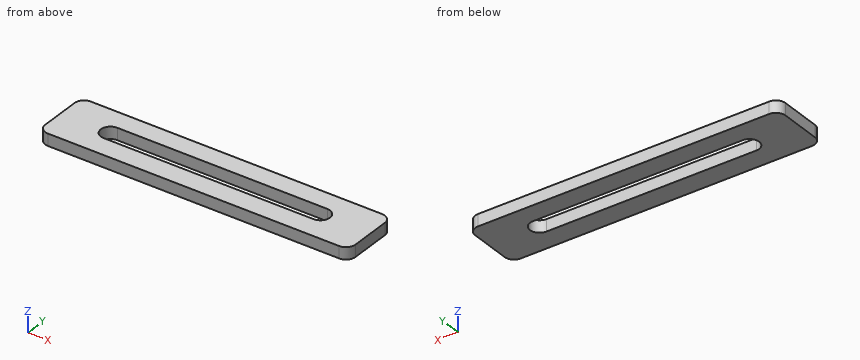
```python
from build123d import *

# Parameters (mm, degrees)
F1_W     = 165.1
F1_H     = 31.75
F2_DEPTH = 6.35
F3_R     = 5.08


# Not quite as in the source:
# - a variable given as a bare number and used for a length is read in inches; the dataset says mm whatever the document's units were


with BuildPart() as f2:
    # F1 (on Top) → F2 (new body)
    with BuildSketch(Plane.XY):
        with Locations((0, -0.3175)):
            Rectangle(F1_W, F1_H)
        with BuildLine():
            ThreePointArc((-55.88, -5.08), (-60.96, 0), (-55.88, 5.08))
            Line((-55.88, 5.08), (0, 5.08))
            Line((0, 5.08), (55.88, 5.08))
            ThreePointArc((55.88, 5.08), (60.96, 0), (55.88, -5.08))
            Line((55.88, -5.08), (0, -5.08))
            Line((0, -5.08), (-55.88, -5.08))
        make_face(mode=Mode.SUBTRACT)
    extrude(amount=F2_DEPTH)

    # F3
    f3_edges = [f2.edges().sort_by_distance(p)[0] for p in [
        (-82.55, 15.5575, 3.175),
        (-82.55, -16.1925, 3.175),
        (82.55, 15.5575, 3.175),
        (82.55, -16.1925, 3.175),
    ]]
    fillet(f3_edges, radius=F3_R)


solid = f2.part
```
Geometry: final body of the model. Coordinates: model frame, mm. Round coordinates to 2 decimals unless told otherwise and drop trailing zeros. Loops run counter-clockwise (first coordinate to the right, second up) from the corner with the lowest first, then second, coordinate; pieces in that order, holes last.
Item 1: Section C-C, the plane z = 4.5. Output: boundary loops of the cut face in (x, y), plus the area to 3 significant figures.
Checked values:
outline: (-82.55, -11.11) arc R5.08 ccw to (-77.47, -16.19) - (77.47, -16.19) arc R5.08 ccw to (82.55, -11.11) - (82.55, 10.48) arc R5.08 ccw to (77.47, 15.56) - (-77.47, 15.56) arc R5.08 ccw to (-82.55, 10.48) - close; hole (-55.88, -5.08) - (55.88, -5.08) arc R5.08 ccw to (55.88, 5.08) - (-55.88, 5.08) arc R5.08 ccw to start
area: 4,000 mm2
Item 2: Line query: L1, parallel to Y at x = 52, z = 1.75; L2, parallel to X at y = 0.5, z = 5; L3, parallel to X at y = 0, z = 1.5. Output: solid intervals per line, ascending.
Checked values:
L1: y = -16.19 to -5.08, 5.08 to 15.56
L2: x = -82.55 to -60.94, 60.94 to 82.55
L3: x = -82.55 to -60.96, 60.96 to 82.55
Item 3: Section A-A, the plane y = 0. Output: boundary loops of the cut face in (x, z), plus the area to 3 significant figures.
Checked values:
outline: (-82.55, 0) - (-60.96, 0) - (-60.96, 6.35) - (-82.55, 6.35) - close; (60.96, 0) - (82.55, 0) - (82.55, 6.35) - (60.96, 6.35) - close
area: 274 mm2
Item 4: Contact query for a flat-ended pin moving along its axis: P1, Ø4, axis at x = 53, y = -4, coming from the -Z side. Output: stop coordinate, or through.
Checked values:
P1: stops at z = 0
Item 5: Section B-B, the plane x = -51.5. Output: boundary loops of the cut face in (y, z).
Checked values:
outline: (-16.19, 0) - (-5.08, 0) - (-5.08, 6.35) - (-16.19, 6.35) - close; (5.08, 0) - (15.56, 0) - (15.56, 6.35) - (5.08, 6.35) - close
